```python
from build123d import *

# Parameters (mm, degrees)
SKETCH_1_W              = 533
SKETCH_1_H              = 398
EXTRUDE_286_DEPTH       = 183
SKETCH_2_R              = 86.5
CUT_EXTRUDE_597_DEPTH   = 81
SKETCH_3_R              = 53
CUT_EXTRUDE_101_DEPTH   = 150
SKETCH_4_R              = 15
CUT_EXTRUDE_1795_DEPTH  = 30
SKETCH_5_W              = 90
SKETCH_5_H              = 35
CUT_EXTRUDE_2164_DEPTH  = 30
CUT_EXTRUDE_597_2_DEPTH = 30


with BuildPart() as part:
    # Эскиз1 → Extrude 286 (new body)
    with BuildSketch(Plane(origin=(0, 0, 0), x_dir=(1, 0, 0), z_dir=(0, 1, 0))):
        with Locations((266.5, 199)):
            Rectangle(SKETCH_1_W, SKETCH_1_H)
    extrude(amount=-EXTRUDE_286_DEPTH)

    # Эскиз2 → Cut-Extrude 597 (cut)
    with BuildSketch(Plane(origin=(0, 0, 0), x_dir=(1, 0, 0), z_dir=(0, 1, 0))):
        with Locations(Location((429.166666667, 103.833333333, 0), (0, 0, 270))):
            Circle(SKETCH_2_R)
        with Locations(Location((238.833333333, 103.833333333, 0), (0, 0, 270))):
            Circle(SKETCH_2_R)
        with Locations(Location((238.833333333, 294.166666667, 0), (0, 0, 270))):
            Circle(SKETCH_2_R)
        with Locations(Location((429.166666667, 294.166666667, 0), (0, 0, 270))):
            Circle(SKETCH_2_R)
    extrude(amount=-CUT_EXTRUDE_597_DEPTH, mode=Mode.SUBTRACT)

    # Эскиз3 → КМЕ-101 (cut)
    with BuildSketch(Plane(origin=(0, 0, 0), x_dir=(1, 0, 0), z_dir=(0, 1, 0))):
        with Locations(Location((81, 283, 0), (0, 0, 270))):
            Circle(SKETCH_3_R)
        with Locations(Location((81, 115, 0), (0, 0, 270))):
            Circle(SKETCH_3_R)
    extrude(amount=-CUT_EXTRUDE_101_DEPTH, mode=Mode.SUBTRACT)

    # Эскиз4 → Cut-Extrude 1795 (cut)
    with BuildSketch(Plane(origin=(0, 0, 0), x_dir=(1, 0, 0), z_dir=(0, 1, 0))):
        with Locations((81, 336)):
            Circle(SKETCH_4_R)
        with Locations((81, 230)):
            Circle(SKETCH_4_R)
        with Locations((81, 168)):
            Circle(SKETCH_4_R)
        with Locations((81, 62)):
            Circle(SKETCH_4_R)
        with Locations((299.998069906, 233.001930094)):
            Circle(SKETCH_4_R)
        with Locations((177.668596761, 355.331403239)):
            Circle(SKETCH_4_R)
        with Locations((368.001930094, 233.001930094)):
            Circle(SKETCH_4_R)
        with Locations((490.331403239, 355.331403239)):
            Circle(SKETCH_4_R)
        with Locations((368.001930094, 164.998069906)):
            Circle(SKETCH_4_R)
        with Locations((490.331403239, 42.668596761)):
            Circle(SKETCH_4_R)
        with Locations((299.998069906, 164.998069906)):
            Circle(SKETCH_4_R)
        with Locations((177.668596761, 42.668596761)):
            Circle(SKETCH_4_R)
    extrude(amount=-CUT_EXTRUDE_1795_DEPTH, mode=Mode.SUBTRACT)

    # Эскиз5 → Cut-Extrude 2164 (cut)
    with BuildSketch(Plane(origin=(0, -81, 0), x_dir=(1, 0, 0), z_dir=(0, 1, 0))):
        with Locations((429.166666667, 294.166666667)):
            Rectangle(SKETCH_5_W, SKETCH_5_H)
        with Locations((238.833333333, 294.166666667)):
            Rectangle(SKETCH_5_W, SKETCH_5_H)
        with Locations((429.166666667, 103.833333333)):
            Rectangle(SKETCH_5_W, SKETCH_5_H)
        with Locations((238.833333333, 103.833333333)):
            Rectangle(SKETCH_5_W, SKETCH_5_H)
    extrude(amount=-CUT_EXTRUDE_2164_DEPTH, mode=Mode.SUBTRACT)

    # Эскиз6 → Cut-Extrude 597 2 (cut)
    with BuildSketch(Plane(origin=(0, -81, 0), x_dir=(1, 0, 0), z_dir=(0, 1, 0))):
        with BuildLine():
            Line((221.333333333, 348.666666667), (256.333333333, 348.666666667))
            ThreePointArc((256.333333333, 348.666666667), (271.333333333, 333.666666667), (256.333333333, 318.666666667))
            Line((256.333333333, 318.666666667), (221.333333333, 318.666666667))
            ThreePointArc((221.333333333, 318.666666667), (206.333333333, 333.666666667), (221.333333333, 348.666666667))
        make_face()
        with BuildLine():
            Line((411.666666667, 348.666666667), (446.666666667, 348.666666667))
            ThreePointArc((446.666666667, 348.666666667), (461.666666667, 333.666666667), (446.666666667, 318.666666667))
            Line((446.666666667, 318.666666667), (411.666666667, 318.666666667))
            ThreePointArc((411.666666667, 318.666666667), (396.666666667, 333.666666667), (411.666666667, 348.666666667))
        make_face()
        with BuildLine():
            Line((411.666666667, 158.333333333), (446.666666667, 158.333333333))
            ThreePointArc((446.666666667, 158.333333333), (461.666666667, 143.333333333), (446.666666667, 128.333333333))
            Line((446.666666667, 128.333333333), (411.666666667, 128.333333333))
            ThreePointArc((411.666666667, 128.333333333), (396.666666667, 143.333333333), (411.666666667, 158.333333333))
        make_face()
        with BuildLine():
            Line((221.333333333, 158.333333333), (256.333333333, 158.333333333))
            ThreePointArc((256.333333333, 158.333333333), (271.333333333, 143.333333333), (256.333333333, 128.333333333))
            Line((256.333333333, 128.333333333), (221.333333333, 128.333333333))
            ThreePointArc((221.333333333, 128.333333333), (206.333333333, 143.333333333), (221.333333333, 158.333333333))
        make_face()
        with BuildLine():
            ThreePointArc((317.469292127, 330.203258966), (313.744530761, 337.416666667), (309.359917127, 344.249108484))
            ThreePointArc((309.359917127, 344.249108484), (300.296811157, 345.785373488), (298.760546153, 336.722267517))
            ThreePointArc((298.760546153, 336.722267517), (302.486200511, 330.916666667), (305.651171153, 324.787354921))
            ThreePointArc((305.651171153, 324.787354921), (314.268183662, 321.586246456), (317.469292127, 330.203258966))
        make_face()
        with BuildLine():
            ThreePointArc((168.306749539, 344.249108484), (163.922135906, 337.416666667), (160.197374539, 330.203258966))
            ThreePointArc((160.197374539, 330.203258966), (163.398483004, 321.586246456), (172.015495514, 324.787354921))
            ThreePointArc((172.015495514, 324.787354921), (175.180466155, 330.916666667), (178.906120514, 336.722267517))
            ThreePointArc((178.906120514, 336.722267517), (177.36985551, 345.785373488), (168.306749539, 344.249108484))
        make_face()
        with BuildLine():
            ThreePointArc((230.723958333, 208.04763255), (238.833333333, 207.666666667), (246.942708333, 208.04763255))
            ThreePointArc((246.942708333, 208.04763255), (252.804705839, 215.128380056), (245.723958333, 220.990377562))
            ThreePointArc((245.723958333, 220.990377562), (238.833333333, 220.666666667), (231.942708333, 220.990377562))
            ThreePointArc((231.942708333, 220.990377562), (224.861960827, 215.128380056), (230.723958333, 208.04763255))
        make_face()
        with BuildLine():
            ThreePointArc((358.640082873, 344.249108484), (354.255469239, 337.416666667), (350.530707873, 330.203258966))
            ThreePointArc((350.530707873, 330.203258966), (353.731816338, 321.586246456), (362.348828847, 324.787354921))
            ThreePointArc((362.348828847, 324.787354921), (365.513799489, 330.916666667), (369.239453847, 336.722267517))
            ThreePointArc((369.239453847, 336.722267517), (367.703188843, 345.785373488), (358.640082873, 344.249108484))
        make_face()
        with BuildLine():
            ThreePointArc((507.802625461, 330.203258966), (504.077864094, 337.416666667), (499.693250461, 344.249108484))
            ThreePointArc((499.693250461, 344.249108484), (490.63014449, 345.785373488), (489.093879486, 336.722267517))
            ThreePointArc((489.093879486, 336.722267517), (492.819533845, 330.916666667), (495.984504486, 324.787354921))
            ThreePointArc((495.984504486, 324.787354921), (504.601516996, 321.586246456), (507.802625461, 330.203258966))
        make_face()
        with BuildLine():
            ThreePointArc((421.057291667, 208.04763255), (429.166666667, 207.666666667), (437.276041667, 208.04763255))
            ThreePointArc((437.276041667, 208.04763255), (443.138039173, 215.128380056), (436.057291667, 220.990377562))
            ThreePointArc((436.057291667, 220.990377562), (429.166666667, 220.666666667), (422.276041667, 220.990377562))
            ThreePointArc((422.276041667, 220.990377562), (415.195294161, 215.128380056), (421.057291667, 208.04763255))
        make_face()
        with BuildLine():
            ThreePointArc((358.640082873, 153.91577515), (354.255469239, 147.083333333), (350.530707873, 139.869925633))
            ThreePointArc((350.530707873, 139.869925633), (353.731816338, 131.252913123), (362.348828847, 134.454021588))
            ThreePointArc((362.348828847, 134.454021588), (365.513799489, 140.583333333), (369.239453847, 146.388934184))
            ThreePointArc((369.239453847, 146.388934184), (367.703188843, 155.452040154), (358.640082873, 153.91577515))
        make_face()
        with BuildLine():
            ThreePointArc((507.802625461, 139.869925633), (504.077864094, 147.083333333), (499.693250461, 153.91577515))
            ThreePointArc((499.693250461, 153.91577515), (490.63014449, 155.452040154), (489.093879486, 146.388934184))
            ThreePointArc((489.093879486, 146.388934184), (492.819533845, 140.583333333), (495.984504486, 134.454021588))
            ThreePointArc((495.984504486, 134.454021588), (504.601516996, 131.252913123), (507.802625461, 139.869925633))
        make_face()
        with BuildLine():
            ThreePointArc((421.057291667, 17.714299217), (429.166666667, 17.333333333), (437.276041667, 17.714299217))
            ThreePointArc((437.276041667, 17.714299217), (443.138039173, 24.795046723), (436.057291667, 30.657044229))
            ThreePointArc((436.057291667, 30.657044229), (429.166666667, 30.333333333), (422.276041667, 30.657044229))
            ThreePointArc((422.276041667, 30.657044229), (415.195294161, 24.795046723), (421.057291667, 17.714299217))
        make_face()
        with BuildLine():
            ThreePointArc((168.306749539, 153.91577515), (163.922135906, 147.083333333), (160.197374539, 139.869925633))
            ThreePointArc((160.197374539, 139.869925633), (163.398483004, 131.252913123), (172.015495514, 134.454021588))
            ThreePointArc((172.015495514, 134.454021588), (175.180466155, 140.583333333), (178.906120514, 146.388934184))
            ThreePointArc((178.906120514, 146.388934184), (177.36985551, 155.452040154), (168.306749539, 153.91577515))
        make_face()
        with BuildLine():
            ThreePointArc((317.469292127, 139.869925633), (313.744530761, 147.083333333), (309.359917127, 153.91577515))
            ThreePointArc((309.359917127, 153.91577515), (300.296811157, 155.452040154), (298.760546153, 146.388934184))
            ThreePointArc((298.760546153, 146.388934184), (302.486200511, 140.583333333), (305.651171153, 134.454021588))
            ThreePointArc((305.651171153, 134.454021588), (314.268183662, 131.252913123), (317.469292127, 139.869925633))
        make_face()
        with BuildLine():
            ThreePointArc((230.723958333, 17.714299217), (238.833333333, 17.333333333), (246.942708333, 17.714299217))
            ThreePointArc((246.942708333, 17.714299217), (252.804705839, 24.795046723), (245.723958333, 30.657044229))
            ThreePointArc((245.723958333, 30.657044229), (238.833333333, 30.333333333), (231.942708333, 30.657044229))
            ThreePointArc((231.942708333, 30.657044229), (224.861960827, 24.795046723), (230.723958333, 17.714299217))
        make_face()
    extrude(amount=-CUT_EXTRUDE_597_2_DEPTH, mode=Mode.SUBTRACT)


solid = part.part
```
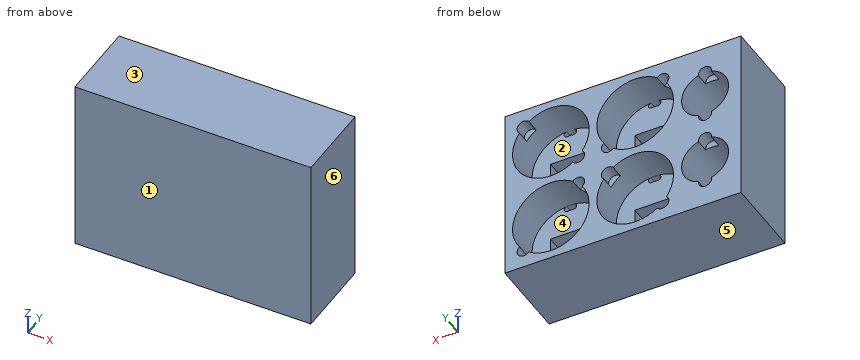
Can you work these out from the model? Positions are in its coordinate system, mm. Face numbers are marked on the shaded views. A direction names the side the tool comes from. Coordinates: 2 decimals unless noted, no trailing zeros. Write each loop counter-clockwise with the first axis right and the second up, starting at its lowest first coordinate (ties: lowest second). Pieces come first, ordered by that corner, then holes. Notation, with made-up numbers: (61.25, 42.25) - (82.25, 42.25) arc R27 ccw to (82.25, 63.25) - close; hole circle Ø7 at (45, 26). An arc over 180 degrees is marked (long way). Return JSON: item names as keys, results as strings.
Q1. Thinking about a two-plate mould opening in Z: for the marked faces 3, 4, 5 and 6, which applies, +Z half, -Z half, draft (parallel to the pull), parting line (faces both ways), or undercut?
Computed values:
{"face 3": "+Z half", "face 4": "undercut", "face 5": "-Z half", "face 6": "draft"}
Q2. Please list where these lines run through material, in increasing order: L1, parallel to X at y = -72, z = -235; L2, parallel to Z at x = 462, y = -83.5; L3, parallel to X at y = -75.5, z = -41. Write a range as from..to.
Computed values:
{"L1": "x = 0..58.53, 103.47..175.73, 301.93..366.07, 492.27..533", "L2": "z = -398..-311.67, -276.67..-121.33, -86.33..0", "L3": "x = 0..179.38, 298.28..369.72, 488.62..533"}
Q3. If we section it at D-D (z = -304.5): Please give me the cut outline in (x, y), then the cut area to 3 significant figures.
Computed values:
{"outline": "(0, -183) - (533, -183) - (533, 0) - (515.05, 0) - (515.05, -81) - (474.17, -81) - (474.17, -111) - (384.17, -111) - (384.17, -81) - (343.29, -81) - (343.29, 0) - (324.71, 0) - (324.71, -81) - (283.83, -81) - (283.83, -111) - (193.83, -111) - (193.83, -81) - (152.95, -81) - (152.95, 0) - (129.44, 0) - (129.44, -150) - (32.56, -150) - (32.56, 0) - (0, 0) - close", "area": "49,800 mm2"}
Q4. If we section it at C-C (y = -57.5): Please give me the cut outline in (x, z), then the cut area to 3 significant figures.
Computed values:
{"outline": "(0, -398) - (533, -398) - (533, 0) - (0, 0) - close; hole circle Ø106 at (81, -283); hole circle Ø106 at (81, -115); hole circle Ø173 at (238.83, -294.17); hole circle Ø173 at (238.83, -103.83); hole circle Ø173 at (429.17, -294.17); hole circle Ø173 at (429.17, -103.83)", "area": "100,000 mm2"}
Q5. If we section it at B-B (x = 81): Please give me the cut outline in (y, z), then the cut area to 3 significant figures.
Computed values:
{"outline": "(-183, -398) - (0, -398) - (0, -351) - (-30, -351) - (-30, -336) - (-150, -336) - (-150, -230) - (-30, -230) - (-30, -215) - (0, -215) - (0, -183) - (-30, -183) - (-30, -168) - (-150, -168) - (-150, -62) - (-30, -62) - (-30, -47) - (0, -47) - (0, 0) - (-183, 0) - close", "area": "39,200 mm2"}
Q6. I'm going to push flat-ended pins straight in: pin 1 Ø9 at (x, y) = (431.5, -90) entering from +Z; pin 2 Ø18 at (x, z) = (300, -165) entering from +Y; pin 3 Ø17.5 at (x, z) = (420, -108.5) entering from +Y. Where does each tip first touch, or does it pass through?
Computed values:
{"pin 1": "stops at z = 0", "pin 2": "stops at y = -30", "pin 3": "stops at y = -111"}
Q7. On a 3-axis mill with a long thin cutter (end or side, diameter ignored), from which of +Z, -Z, +X, -X, +Y, -Y can I reach the whole of each face in a straight line? I mean the marked faces 1 and 2. Say none if no direction works.
Computed values:
{"face 1": "+Z, -Z, +X, -X, -Y", "face 2": "+Y"}
Q8. If we section it at A-A (y = -138.5): Please give me the cut outline in (x, z).
Computed values:
{"outline": "(0, -398) - (533, -398) - (533, 0) - (0, 0) - close; hole circle Ø106 at (81, -283); hole circle Ø106 at (81, -115)"}
